Here's the drawing with two shaded views (mm, measured from the low corner). I have some questions. Round coordinates to 2 decimals unless told otherwise and drop trailing zeros. Order: outer loops, then holes, each group sorted by start corner. A loop starts at its lowest first (then second) coordinate and runs counter-clockwise, first axis right, second up.
Q1. If I drill on line 1 (X direction, y = 4.5, z = 0.35); line 2 (X direction, y = 2, z = 1); line 3 (Y direction, x = 63, z = 1.75), over which ranges is the centre line in solid material (lowest first)?
Q2. If we section it at A-A (z = 1.5): Please give me the cut outline in (x, y).
Q3. If we section it at B-B (y = 8): Please give me the cut outline in (x, z), plus the area to 3 significant figures.
Q4. Will this pin go through, and if not, where does the flat tip stop? P1, Ø0.5, axis at y = 4, z = 1.5, coming from the -X side.
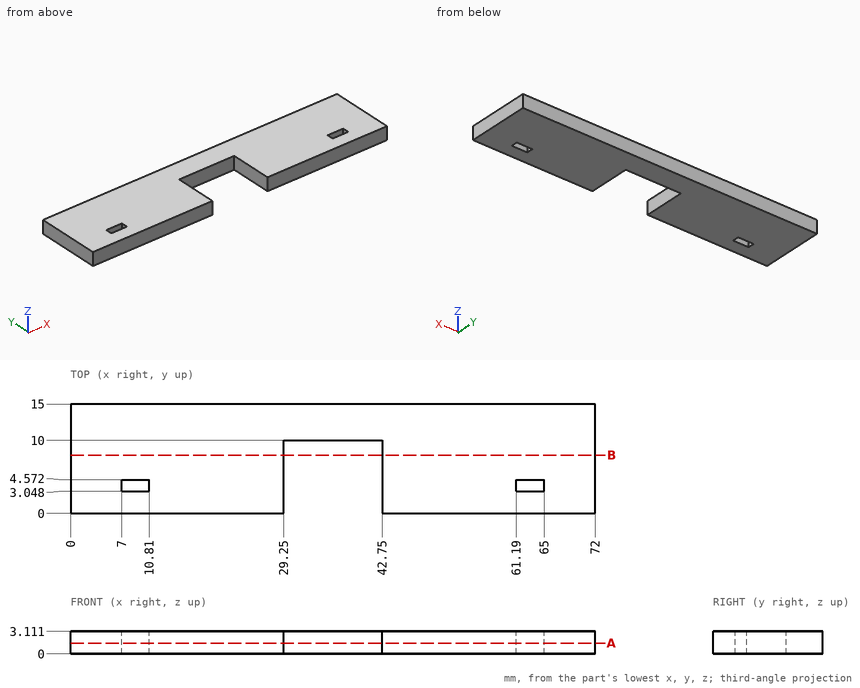
Solution:
1. line 1: x = 0 to 7, 10.81 to 29.25, 42.75 to 61.19, 65 to 72
1. line 2: x = 0 to 29.25, 42.75 to 72
1. line 3: y = 0 to 3.05, 4.57 to 15
2. outline: (0, 0) - (29.25, 0) - (29.25, 10) - (42.75, 10) - (42.75, 0) - (72, 0) - (72, 15) - (0, 15) - close; hole (7, 3.05) - (10.81, 3.05) - (10.81, 4.57) - (7, 4.57) - close; hole (61.19, 3.05) - (65, 3.05) - (65, 4.57) - (61.19, 4.57) - close
3. outline: (0, 0) - (29.25, 0) - (29.25, 3.11) - (0, 3.11) - close; (42.75, 0) - (72, 0) - (72, 3.11) - (42.75, 3.11) - close
3. area: 182 mm2
4. P1: stops at x = 0
